```python
from build123d import *

# Parameters (mm, degrees)
SKETCH_1_W                     = 370
SKETCH_1_H                     = 320
EXTRUDE_1_DEPTH                = 20
SKETCH_2_W                     = 3
SKETCH_2_H                     = 83.6
CUT_EXTRUDE_1_DEPTH            = 490.591666596
SKETCH_3_W                     = 90
SKETCH_3_H                     = 2
CUT_EXTRUDE_2_DEPTH            = 490.591666596
SKETCH_4_W                     = 20
SKETCH_4_H                     = 2
CUT_EXTRUDE_3_DEPTH            = 490.591666596
SKETCH_6_W                     = 90
SKETCH_6_H                     = 320
EXTRUDE_2_DEPTH                = 2
SKETCH_5_W                     = 2
SKETCH_5_H                     = 15
CUT_EXTRUDE_4_DEPTH            = 490.591666596
SKETCH_7_R                     = 2.5
CUT_EXTRUDE_5_DEPTH            = 15
HOLE_WIZARD_M6_1_D             = 5
HOLE_WIZARD_M6_1_DEPTH         = 15
HOLE_WIZARD_M6_1_TIP           = 1.502151548
SKETCH_10_R                    = 2.5
CUT_EXTRUDE_6_DEPTH            = 15
HOLE_WIZARD_M6_2_D             = 5
HOLE_WIZARD_M6_2_DEPTH         = 15
HOLE_WIZARD_M6_2_TIP           = 1.502151548
SKETCH_13_R                    = 3
CUT_EXTRUDE_7_DEPTH            = 490.591666596
HOLE_WIZARD_M6_3_D             = 5
HOLE_WIZARD_M6_3_DEPTH         = 15
HOLE_WIZARD_M6_3_TIP           = 1.502151548
HOLE_WIZARD_M3_1_D             = 3.6
HOLE_WIZARD_M3_1_CBORE_D       = 6.5
HOLE_WIZARD_M3_1_CBORE_DEPTH   = 3
HOLE_WIZARD_M3_2_D             = 3.6
HOLE_WIZARD_M3_2_CBORE_D       = 6.5
HOLE_WIZARD_M3_2_CBORE_DEPTH   = 3
HOLE_WIZARD_M5_1_D             = 4.2
HOLE_WIZARD_M5_1_DEPTH         = 12.4
HOLE_WIZARD_M5_1_TIP           = 1.2618073
HOLE_WIZARD_M4_2_D             = 3.3
HOLE_WIZARD_M4_2_DEPTH         = 10.1
HOLE_WIZARD_M4_2_TIP           = 0.991420021
HOLE_WIZARD_M4_3_D             = 3.3
HOLE_WIZARD_M4_3_DEPTH         = 10.1
HOLE_WIZARD_M4_3_TIP           = 0.991420021
HOLE_WIZARD_M5_2_D             = 4.2
HOLE_WIZARD_M5_2_DEPTH         = 12.4
HOLE_WIZARD_M5_2_TIP           = 1.2618073
SKETCH_30_W                    = 15.1
SKETCH_30_H                    = 3
CUT_EXTRUDE_8_DEPTH            = 440.528110591
HOLE_WIZARD_M6_1_2_D           = 6.6
HOLE_WIZARD_M6_1_2_CBORE_D     = 11
HOLE_WIZARD_M6_1_2_CBORE_DEPTH = 6


with BuildPart() as part:
    # 草图1 → 凸台-拉伸1 (new body)
    with BuildSketch(Plane.XY):
        with Locations((185, 160)):
            Rectangle(SKETCH_1_W, SKETCH_1_H)
    extrude(amount=EXTRUDE_1_DEPTH)

    # 草图2 → 切除-拉伸1 (cut, through all)
    with BuildSketch(Plane(origin=(370, 0, 0), x_dir=(0, 0, -1), z_dir=(1, 0, 0))):
        with Locations((-1.5, 41.8)):
            Rectangle(SKETCH_2_W, SKETCH_2_H)
        with Locations((-1.5, 278.2)):
            Rectangle(SKETCH_2_W, SKETCH_2_H)
    extrude(amount=-CUT_EXTRUDE_1_DEPTH, mode=Mode.SUBTRACT)

    # 草图3 → 切除-拉伸2 (cut, through all)
    with BuildSketch(Plane.XZ):
        with Locations((185, 19)):
            Rectangle(SKETCH_3_W, SKETCH_3_H)
    extrude(amount=-CUT_EXTRUDE_2_DEPTH, mode=Mode.SUBTRACT)

    # 草图4 → 切除-拉伸3 (cut, through all)
    with BuildSketch(Plane.XZ):
        with Locations((80, 19)):
            Rectangle(SKETCH_4_W, SKETCH_4_H)
        with Locations((290, 19)):
            Rectangle(SKETCH_4_W, SKETCH_4_H)
    extrude(amount=-CUT_EXTRUDE_3_DEPTH, mode=Mode.SUBTRACT)

    # 草图6 → 凸台-拉伸2 (add)
    with BuildSketch(Plane.XY.offset(18)):
        with Locations((185, 160)):
            Rectangle(SKETCH_6_W, SKETCH_6_H)
    extrude(amount=EXTRUDE_2_DEPTH)

    # 草图5 → 切除-拉伸4 (cut, through all)
    with BuildSketch(Plane(origin=(370, 0, 0), x_dir=(0, 0, -1), z_dir=(1, 0, 0))):
        with Locations((-1, 160)):
            Rectangle(SKETCH_5_W, SKETCH_5_H)
    extrude(amount=-CUT_EXTRUDE_4_DEPTH, mode=Mode.SUBTRACT)

    # 草图7 → 切除-拉伸5 (cut)
    with BuildSketch(Plane.ZY):
        with Locations((10, 145)):
            Circle(SKETCH_7_R)
    extrude(amount=-CUT_EXTRUDE_5_DEPTH, mode=Mode.SUBTRACT)

    # Hole Wizard M6 _1
    with Locations(Plane.XY.offset(20)):
        with Locations((5, 145)):
            Hole(HOLE_WIZARD_M6_1_D / 2, depth=HOLE_WIZARD_M6_1_DEPTH)
            with Locations((0, 0, -(HOLE_WIZARD_M6_1_DEPTH + HOLE_WIZARD_M6_1_TIP / 2))):  # 118° drill point
                Cone(0, HOLE_WIZARD_M6_1_D / 2, HOLE_WIZARD_M6_1_TIP, mode=Mode.SUBTRACT)

    # 草图10 → 切除-拉伸6 (cut)
    with BuildSketch(Plane(origin=(370, 0, 0), x_dir=(0, 0, -1), z_dir=(1, 0, 0))):
        with Locations((-10, 120)):
            Circle(SKETCH_10_R)
    extrude(amount=-CUT_EXTRUDE_6_DEPTH, mode=Mode.SUBTRACT)

    # M6 螺纹孔2
    with Locations(Plane.XY.offset(20)):
        with Locations((365, 120)):
            Hole(HOLE_WIZARD_M6_2_D / 2, depth=HOLE_WIZARD_M6_2_DEPTH)
            with Locations((0, 0, -(HOLE_WIZARD_M6_2_DEPTH + HOLE_WIZARD_M6_2_TIP / 2))):  # 118° drill point
                Cone(0, HOLE_WIZARD_M6_2_D / 2, HOLE_WIZARD_M6_2_TIP, mode=Mode.SUBTRACT)

    # 草图13 → 切除-拉伸7 (cut, through all)
    with BuildSketch(Plane.XY.offset(20)):
        with Locations((210, 40)):
            Circle(SKETCH_13_R)
        with Locations((160, 290)):
            Circle(SKETCH_13_R)
    extrude(amount=-CUT_EXTRUDE_7_DEPTH, mode=Mode.SUBTRACT)

    # M6 螺纹孔3
    with Locations(Plane.XY.offset(20)):
        with Locations((160, 70), (210, 70), (160, 250), (210, 250), (290, 25), (290, 160), (290, 295), (80, 295), (80, 160), (80, 25)):
            Hole(HOLE_WIZARD_M6_3_D / 2, depth=HOLE_WIZARD_M6_3_DEPTH)
            with Locations((0, 0, -(HOLE_WIZARD_M6_3_DEPTH + HOLE_WIZARD_M6_3_TIP / 2))):  # 118° drill point
                Cone(0, HOLE_WIZARD_M6_3_D / 2, HOLE_WIZARD_M6_3_TIP, mode=Mode.SUBTRACT)

    # M3 六角凹头螺钉的柱形沉头孔1 (through all)
    with Locations(Plane.XY.offset(20)):
        with Locations((270, 80), (250, 60), (250, 80), (270, 60), (120, 60), (100, 60), (100, 80), (120, 80)):
            CounterBoreHole(HOLE_WIZARD_M3_1_D / 2, HOLE_WIZARD_M3_1_CBORE_D / 2, HOLE_WIZARD_M3_1_CBORE_DEPTH)

    # M3 六角凹头螺钉的柱形沉头孔2 (through all)
    with Locations(Plane.XY.offset(20)):
        with Locations((100, 260), (270, 260), (250, 260), (250, 240), (270, 240), (120, 260), (100, 240), (120, 240)):
            CounterBoreHole(HOLE_WIZARD_M3_2_D / 2, HOLE_WIZARD_M3_2_CBORE_D / 2, HOLE_WIZARD_M3_2_CBORE_DEPTH)

    # M5 螺纹孔1
    with Locations(Plane(origin=(0, 0, 2), x_dir=(-1, 0, 0), z_dir=(0, 0, -1))):
        with Locations((-264, 160), (-183, 160), (-21, 160), (-102, 160)):
            Hole(HOLE_WIZARD_M5_1_D / 2, depth=HOLE_WIZARD_M5_1_DEPTH)
            with Locations((0, 0, -(HOLE_WIZARD_M5_1_DEPTH + HOLE_WIZARD_M5_1_TIP / 2))):  # 118° drill point
                Cone(0, HOLE_WIZARD_M5_1_D / 2, HOLE_WIZARD_M5_1_TIP, mode=Mode.SUBTRACT)

    # M4 螺纹孔2
    with Locations(Plane(origin=(0, 0, 0), x_dir=(-1, 0, 0), z_dir=(0, 0, -1))):
        with Locations((-117, 220.5), (-127, 220.5), (-244, 220.5), (-254, 220.5)):
            Hole(HOLE_WIZARD_M4_2_D / 2, depth=HOLE_WIZARD_M4_2_DEPTH)
            with Locations((0, 0, -(HOLE_WIZARD_M4_2_DEPTH + HOLE_WIZARD_M4_2_TIP / 2))):  # 118° drill point
                Cone(0, HOLE_WIZARD_M4_2_D / 2, HOLE_WIZARD_M4_2_TIP, mode=Mode.SUBTRACT)

    # M4 螺纹孔3
    with Locations(Plane(origin=(0, 0, 3), x_dir=(-1, 0, 0), z_dir=(0, 0, -1))):
        with Locations((-253, 40.5), (-243, 40.5), (-128, 40.5), (-118, 40.5)):
            Hole(HOLE_WIZARD_M4_3_D / 2, depth=HOLE_WIZARD_M4_3_DEPTH)
            with Locations((0, 0, -(HOLE_WIZARD_M4_3_DEPTH + HOLE_WIZARD_M4_3_TIP / 2))):  # 118° drill point
                Cone(0, HOLE_WIZARD_M4_3_D / 2, HOLE_WIZARD_M4_3_TIP, mode=Mode.SUBTRACT)

    # M5 螺纹孔2
    with Locations(Plane.XY.offset(20)):
        with Locations((348, 80), (348, 170)):
            Hole(HOLE_WIZARD_M5_2_D / 2, depth=HOLE_WIZARD_M5_2_DEPTH)
            with Locations((0, 0, -(HOLE_WIZARD_M5_2_DEPTH + HOLE_WIZARD_M5_2_TIP / 2))):  # 118° drill point
                Cone(0, HOLE_WIZARD_M5_2_D / 2, HOLE_WIZARD_M5_2_TIP, mode=Mode.SUBTRACT)

    # 草图30 → 切除-拉伸8 (cut, through all)
    with BuildSketch(Plane.XZ.offset(-83.6)):
        with Locations((117.55, 1.5)):
            Rectangle(SKETCH_30_W, SKETCH_30_H)
    extrude(amount=-CUT_EXTRUDE_8_DEPTH, mode=Mode.SUBTRACT)

    # Hole Wizard M6 _1 2 (through all)
    with Locations(Plane.XY.offset(20)):
        with Locations((117.55, 137), (117.55, 183)):
            CounterBoreHole(HOLE_WIZARD_M6_1_2_D / 2, HOLE_WIZARD_M6_1_2_CBORE_D / 2, HOLE_WIZARD_M6_1_2_CBORE_DEPTH)


solid = part.part
```
Verification items for the finished model (mm, model axes). A direction names the side the tool comes from. Coordinates: 2 decimals unless noted, no trailing zeros. Write each loop counter-clockwise with the first axis right and the second up, starting at its lowest first coordinate (ties: lowest second). Pieces come first, ordered by that corner, then holes. Notation, with made-up numbers: (60.5, -33) - (100.5, -33) arc R16 cw to (100.5, -10) - close; hole circle Ø9 at (64, 8.25). An arc over 180 degrees is marked (long way). One line per question, with ' | ' between items. Start each with the question number.
1. Access from +Z, -Z, +X, -X, +Y, -Y to the whole of each face (thin tool, end or side, straight path). Record for faces 1 (the cylindrical face through (122.63, 180.89, 17.04)), 2 (the flat face through (288, 158, 18)), 3 (the flat face through (0, 158, 10)), 4 (the flat face through (249, 160, 2)).
2. Draft check along Y on faces 5 (the flat face through (182, 320, 11)), 6 (the flat face through (54, 119, 0)), 7 (the flat face through (56, 160, 2)). Enter one of: released by +Y, released by -Y, zero draft, split by the parting line, or undercut.
3. Gauge pin test, flat ends, axial feed: P1, Ø2, axis at x = 270.5, y = 241.5, coming from the +Z side; P2, Ø8, axis at x = 290, y = 25, coming from the +Z side; P3, Ø6, axis at x = 80, y = 295, coming from the -Z side; P4, Ø3, axis at x = 250, y = 60, coming from the -Z side. Record the tip position at first contact, or that the pin passes through.
4. Material ranges on line 1 along Y through (x, z) = (270, 19.15); line 2 along Y through (x, z) = (117.5, 8.5); line 3 along X through (y, z) = (40.5, 10.25), recorded low to high.
5. Section check A-A (x = 312). Enter the section's corners in (y, z).
Computed values:
1) face 1: +Z | face 2: +Z, +Y, -Y | face 3: +Z, -Z, -X, +Y, -Y | face 4: -Z, +X, -X
2) face 5: released by +Y | face 6: zero draft | face 7: undercut
3) P1: z = 17 | P2: z = 18 | P3: z = 3 | P4: through
4) line 1: 0 to 56.75, 63.25 to 76.75, 83.25 to 236.75, 243.25 to 256.75, 263.25 to 320 | line 2: 0 to 38.93, 42.07 to 133.7, 140.3 to 179.7, 186.3 to 218.93, 222.07 to 320 | line 3: 0 to 116.35, 119.65 to 126.35, 129.65 to 207.04, 212.96 to 241.35, 244.65 to 251.35, 254.65 to 370
5) outline: (0, 3) - (83.6, 3) - (83.6, 0) - (152.5, 0) - (152.5, 2) - (167.5, 2) - (167.5, 0) - (236.4, 0) - (236.4, 3) - (320, 3) - (320, 20) - (0, 20) - close
